Design review of the part built by this model. Coordinates are the model's own, in mm. Face numbers are marked on the shaded views. Coordinates: 2 decimals unless noted, no trailing zeros. Write each loop counter-clockwise with the first axis right and the second up, starting at its lowest first coordinate (ties: lowest second). Pieces come first, ordered by that corner, then holes.
Q1. Insertion check: pin 1 (1 mm diameter, centred on x = -2, z = -0.5, fed in from -Y); pin 2 (2 mm diameter, centred on x = 0, z = -1, fed in from -Y). Each pin has a flat end and moves straight along its axis. Give the tip position at first contact, or say it passes through.
Q2. Take a section at A-A (z = 0). Give the boundary of the cut face in (x, y), and give its area (3 significant figures).
Q3. For probe 1 along Z at (x, y) = (0, -0.7); probe 2 along Y at (x, z) = (-2, 0.5); probe 3 along Y at (x, z) = (0.75, -4), list the stretches that pass through material, from the lowest coordinate up.
Q4. Mouldability with a two-part tool opening along X and no side actions: class the marked faces 1, 2, 3 and 4 as pulls with the +X half, pulls with the -X half, needs draft (parallel to the pull), parting line crosses it, or undercut.
Q5. Take a section at D-D (y = 2.25). Give the boundary of the cut face in (x, z), and give its area (3 significant figures).
Q6. Take a section at C-C (y = -0.65). Give the boundary of the cut face in (x, z).
Q7. Take a section at B-B (x = 0). Give the boundary of the cut face in (y, z), and give its area (3 significant figures).
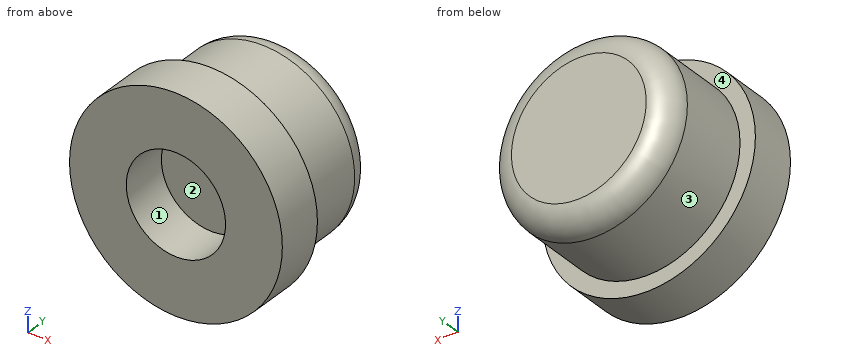
Autodesk Inventor part; units mm, degrees
ref_plane "YZ Plane" through (0, 0, 0) normal (1, 0, 0) x (0, 1, 0)
ref_plane "XZ Plane" through (0, 0, 0) normal (0, 1, 0) x (-1, 0, 0)
ref_plane "XY Plane" through (0, 0, 0) normal (0, 0, 1) x (1, 0, 0)
sketch "Sketch1" plane through (0, 0, 0) normal (0, 1, 0) x (-1, 0, 0)
  circle A0 centre (0, 0) radius 3.85
  dimension "d0" = 7.7
extrude "Extrusion1" add sketch "Sketch1" along normal blind 4
fillet "Fillet1" radius 1 1 edges at (3.85, 4, 0)
sketch "Sketch2" plane through (0, 0, 0) normal (0, -1, 0) x (1, 0, 0)
  circle A0 centre (0, 0) radius 4.5
  dimension "d4" = 9
extrude "Extrusion2" add sketch "Sketch2" along normal blind 2
sketch "Sketch3" plane through (0, -2, 0) normal (0, -1, 0) x (1, 0, 0)
  circle A0 centre (0, 0) radius 2.1
  dimension "d7" = 4.2
extrude "Extrusion3" cut sketch "Sketch3" against normal blind 2
properties part number "tlacitko"
Response:
1. pin 1: stops at y = -2
1. pin 2: stops at y = 0
2. outline: (-4.5, -2) - (-2.1, -2) - (-2.1, 0) - (2.1, 0) - (2.1, -2) - (4.5, -2) - (4.5, 0) - (3.85, 0) - (3.85, 3) arc R1 ccw to (2.85, 4) - (-2.85, 4) arc R1 ccw to (-3.85, 3) - (-3.85, 0) - (-4.5, 0) - close
2. area: 40.0 mm2
3. probe 1: z = -4.5 to -2.1, 2.1 to 4.5
3. probe 2: y = 0 to 4
3. probe 3: y = -2 to 0
4. face 1: undercut
4. face 2: undercut
4. face 3: parting line crosses it
4. face 4: needs draft
5. outline: circle Ø7.7 at (0, 0)
5. area: 46.6 mm2
6. outline: circle Ø9 at (0, 0); hole circle Ø4.2 at (0, 0)
7. outline: (-2, -4.5) - (0, -4.5) - (0, -3.85) - (3, -3.85) arc R1 ccw to (4, -2.85) - (4, 2.85) arc R1 ccw to (3, 3.85) - (0, 3.85) - (0, 4.5) - (-2, 4.5) - (-2, 2.1) - (0, 2.1) - (0, -2.1) - (-2, -2.1) - close
7. area: 40.0 mm2
